from build123d import *

# Parameters (mm, degrees)
ESBO_O1_W                = 9.773502692
ESBO_O1_H                = 9.773502692
RESSALTO_EXTRUS_O1_DEPTH = 3


with BuildPart() as part:
    # Esboço1 → Ressalto-extrusão1 (new body)
    with BuildSketch(Plane(origin=(0, 0, 0), x_dir=(1, 0, 0), z_dir=(0, 1, 0))):
        Rectangle(ESBO_O1_W, ESBO_O1_H)
        Polygon((1.443375673, 2.5), (-1.443375673, 2.5), (-2.886751346, 0), (-1.443375673, -2.5), (1.443375673, -2.5), (2.886751346, 0), align=None, mode=Mode.SUBTRACT)
    extrude(amount=RESSALTO_EXTRUS_O1_DEPTH)


solid = part.part
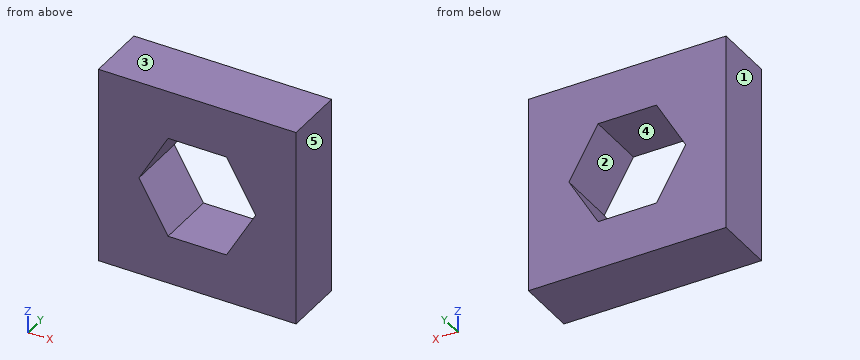
CAD build for the part. Positions are in the model's coordinates, mm. Face numbers are marked on the shaded views. A direction names the side the tool comes from. Give positions to 0.01 mm unless a question says otherwise; leave off trailing zeros. Loops run counter-clockwise (first coordinate to the right, second up) from the corner with the lowest first, then second, coordinate; pieces in that order, holes last. Notation, with made-up numbers: M -14,59.5 L 26,59.5 A27 ccw 26,92.5 Z; hole C 88.25,37 d7. An arc over 180 degrees is marked long. Write each question's results on one line, items separated by ' | '.
Q1. Mould opens along X. For the marked faces 3, 4 and 5 say: pulls with the +X half, pulls with the -X half, needs draft (parallel to the pull), parting line crosses it, or undercut.
Geometry check:
face 3: needs draft | face 4: undercut | face 5: pulls with the +X half
Q2. Band-saw the part on B-B on z = -1.5. Write the cut outline in (x, y), and give its area (3 significant figures).
Geometry check:
outline: M -4.89,0 L -2.02,0 L -2.02,3 L -4.89,3 Z; M 2.02,0 L 4.89,0 L 4.89,3 L 2.02,3 Z | area: 17.2 mm²
Q3. Band-saw the part on C-C on y = 0.5. Write the cut outline in (x, z).
Geometry check:
outline: M -4.89,-4.89 L 4.89,-4.89 L 4.89,4.89 L -4.89,4.89 Z; hole M -2.89,0 L -1.44,-2.5 L 1.44,-2.5 L 2.89,0 L 1.44,2.5 L -1.44,2.5 Z
Q4. Band-saw the part on A-A on x = -0.5. Write the cut outline in (y, z), and give its area (3 significant figures).
Geometry check:
outline: M 0,-4.89 L 3,-4.89 L 3,-2.5 L 0,-2.5 Z; M 0,2.5 L 3,2.5 L 3,4.89 L 0,4.89 Z | area: 14.3 mm²
Q5. Probe probe 1 along Z at (x, y) = (0.5, 0.8); probe 2 along X at (y, z) = (1.2, -1.75); probe 3 along X at (y, z) = (1.7, -1.5). List the from-to ranges inside material, lowest first.
Geometry check:
probe 1: z = -4.89 to -2.5, 2.5 to 4.89 | probe 2: x = -4.89 to -1.88, 1.88 to 4.89 | probe 3: x = -4.89 to -2.02, 2.02 to 4.89
Q6. Which spindle directions (+Z, -Z, +X, -X, +Y, -Y) get a long thin tool onto all of the face, cutting with end or side? Do the marked faces 1 and 2. Say none if no direction does.
Geometry check:
face 1: +Z, -Z, -X, +Y, -Y | face 2: +Y, -Y
